from build123d import *

# Parameters (mm, degrees)
SKETCH1_W               = 12
SKETCH1_H               = 7
BOSS_EXTRUDE1_DEPTH     = 3
CUT_EXTRUDE1_DEPTH      = 7
CUT_EXTRUDE2_DEPTH      = 15.212670404
CUT_EXTRUDE2_DEPTH_BACK = 15.212670404
SKETCH4_R               = 1.8
CUT_EXTRUDE3_DEPTH      = 0.8
CUT_EXTRUDE4_DEPTH      = 0.4


with BuildPart() as part:
    # Sketch1 → Boss-Extrude1 (new body)
    with BuildSketch(Plane(origin=(0, 0, 0), x_dir=(1, 0, 0), z_dir=(0, 1, 0))):
        with Locations((6, 3.5)):
            Rectangle(SKETCH1_W, SKETCH1_H)
    extrude(amount=BOSS_EXTRUDE1_DEPTH)

    # Sketch2 → Cut-Extrude1 (cut)
    with BuildSketch(Plane.XY):
        Polygon((0, 0), (0.7, 3), (0, 3), align=None)
        Polygon((12, 0), (11.3, 3), (12, 3), align=None)
    extrude(amount=-CUT_EXTRUDE1_DEPTH, mode=Mode.SUBTRACT)

    # Sketch3 → Cut-Extrude2 (cut, two sides: drawn at the far end of the back side and taken through both)
    with BuildSketch(Plane(origin=(0, 0, 0), x_dir=(0, 0, -1), z_dir=(1, 0, 0)).offset(-CUT_EXTRUDE2_DEPTH_BACK)):
        Polygon((0, 0), (0.7, 3), (0, 3), align=None)
        Polygon((7, 3), (6.3, 3), (7, 0), align=None)
    extrude(amount=CUT_EXTRUDE2_DEPTH + CUT_EXTRUDE2_DEPTH_BACK, mode=Mode.SUBTRACT)

    # Sketch4 → Cut-Extrude3 (cut)
    with BuildSketch(Plane.XZ):
        with Locations(Location((6, -3.5, 0), (0, 0, 270))):
            Circle(SKETCH4_R)
    extrude(amount=-CUT_EXTRUDE3_DEPTH, mode=Mode.SUBTRACT)

    # Sketch5 → Cut-Extrude4 (cut)
    # profile 1 of 3: a face of its own
    with BuildSketch(Plane(origin=(0, 3, 0), x_dir=(1, 0, 0), z_dir=(0, 1, 0))):
        Polygon((4.994280794, 2.275548034), (4.443679833, 2.275548034), (4.215975506, 2.898624958), (3.179677429, 2.898624958), (2.951973102, 2.275548034), (2.398126948, 2.275548034), (3.418739929, 4.975548034), (3.968800025, 4.975548034), align=None)
        Polygon((4.051011564, 3.348624958), (3.696203871, 4.317855727), (3.34247791, 3.348624958), align=None, mode=Mode.SUBTRACT)
    # profile 2 of 3: a face of its own
    with BuildSketch(Plane(origin=(0, 3, 0), x_dir=(1, 0, 0), z_dir=(0, 1, 0))):
        Polygon((5.271203871, 2.275548034), (5.271203871, 4.975548034), (5.79043464, 4.975548034), (5.79043464, 2.725548034), (7.175050025, 2.725548034), (7.175050025, 2.275548034), align=None)
    # profile 3 of 3: a face of its own
    with BuildSketch(Plane(origin=(0, 3, 0), x_dir=(1, 0, 0), z_dir=(0, 1, 0))):
        Polygon((8.178896179, 2.275548034), (8.178896179, 4.525548034), (7.382742333, 4.525548034), (7.382742333, 4.975548034), (9.494280794, 4.975548034), (9.494280794, 4.525548034), (8.698126948, 4.525548034), (8.698126948, 2.275548034), align=None)
    extrude(amount=-CUT_EXTRUDE4_DEPTH, mode=Mode.SUBTRACT)


solid = part.part
For this review, take the finished solid that the model builds, in its own axes (mm). A direction names the side the tool comes from. Round coordinates to 2 decimals unless told otherwise and drop trailing zeros. Loops run counter-clockwise (first coordinate to the right, second up) from the corner with the lowest first, then second, coordinate; pieces in that order, holes last. Notation, with made-up numbers: (1, -0.5) - (26, -0.5) arc R27 ccw to (26, 30.5) - close; hole circle Ø6 at (85.5, 81.25). An arc over 180 degrees is marked (long way). Put each result on its own line as item: value. Start each with the question number.
1. Consider section B-B on z = -3.5. State the section outline as (x, y) points, plus the area to 3 significant figures.
2. Consider section C-C on y = 0.4. State the section outline as (x, z) points.
3. For probe 1 along Z at (x, y) = (6.75, 2.75); probe 2 along Y at (x, z) = (7.25, -2.25); probe 3 along X at (y, z) = (0.55, -3.5), list the stretches that pass through material, from the lowest coordinate up. Write a range as [from, to].
4. Mouldability with a two-part tool opening along Z and no side actions: class faces 1 (the cylindrical face through (4.403, 0.394, -4.331)), 2 (the flat face through (6, 3, -4)), 3 (the flat face through (5.916, 1.479, -0.345)), 4 (the flat face through (2.9, 2.8, -3.6)) as +Z half, -Z half, draft (parallel to the pull), parting line (faces both ways), or undercut.
5. For faces 5 (the flat face through (5.916, 1.521, -6.645)), 6 (the flat face through (4.474, 2.803, -3.644)), 7 (the flat face through (6, 0.8, -3)), list the 3-axis set-ups (+Z, -Z, +X, -X, +Y, -Y) from which the entire face can be reached by the end or side of a thin tool; tool diameter is ignored.
6. Consider section D-D on y = 2.4. State the section outline as (x, z) points.
7. Insertion check: P1, Ø1.5, axis at x = 1.5, y = 2, coming from the +Z side. The pin has a flat end and moves straight along its axis. Give the tip position at first contact, or say it passes through.
8. Consider section A-A on x = 6. State the section outline as (y, z) points, plus the area to 3 significant figures.
Result sheet:
1. outline: (0, 0) - (4.2, 0) - (4.2, 0.8) - (7.8, 0.8) - (7.8, 0) - (12, 0) - (11.3, 3) - (8.7, 3) - (8.7, 2.6) - (8.18, 2.6) - (8.18, 3) - (5.79, 3) - (5.79, 2.6) - (5.27, 2.6) - (5.27, 3) - (4.53, 3) - (4.53, 2.6) - (4, 2.6) - (4, 3) - (3.4, 3) - (3.4, 2.6) - (2.86, 2.6) - (2.86, 3) - (0.7, 3) - close
1. area: 30.2 mm^2
2. outline: (0.09, -6.91) - (11.91, -6.91) - (11.91, -0.09) - (0.09, -0.09) - close; hole circle Ø3.6 at (6, -3.5)
3. probe 1: [-6.36, -2.73], [-2.28, -0.64]
3. probe 2: [0.8, 3]
3. probe 3: [0.13, 4.2], [7.8, 11.87]
4. face 1: undercut
4. face 2: draft
4. face 3: +Z half
4. face 4: undercut
5. face 5: -Z, +X, -X, +Y
5. face 6: +Y
5. face 7: -Y
6. outline: (0.56, -6.44) - (11.44, -6.44) - (11.44, -0.56) - (0.56, -0.56) - close
7. P1: z = -0.29
8. outline: (0, -7) - (3, -6.3) - (3, -2.73) - (2.6, -2.73) - (2.6, -2.28) - (3, -2.28) - (3, -0.7) - (0, 0) - (0, -1.7) - (0.8, -1.7) - (0.8, -5.3) - (0, -5.3) - close
8. area: 15.8 mm^2
